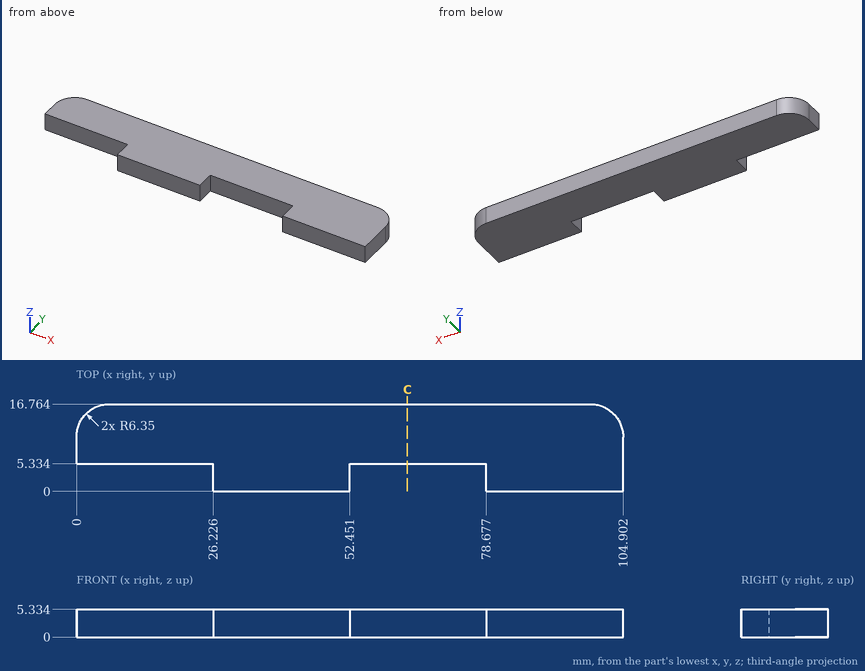
Geometry check sheet. Reference: drawing and pictorial views, mm from the part's lowest x, y, z. Round coordinates to 2 decimals unless told otherwise and drop trailing zeros. Order: outer loops, then holes, each group sorted by start corner. A loop starts at its lowest first (then second) coordinate and runs counter-clockwise, first axis right, second up. Notation, with made-up numbers: (-38.75, -33) - (-33.75, -33) arc R22 cw to (-33.75, -22) - close; hole circle Ø5 at (79.5, -6). An arc over 180 degrees is marked (long way). Use a Markdown table: item, result. Add a question column.
1) Gauge pin test, flat ends, axial feed: P1, Ø2, axis at x = 74.5, z = 1.5, coming from the -Y side; P2, Ø2, axis at y = 14, z = 4, coming from the +X side; P3, Ø2.5, axis at y = 2.5, z = 2.5, coming from the -X side (1 decimal). Record the tip position at first contact, or that the pin passes through.
2) Thickness scan on line 1 along Y through (x, z) = (76.5, 4.6) (1 decimal); line 2 along X through (y, z) = (15.25, 4.7) (1 decimal); line 3 along Y through (x, z) = (5.5, 4.2) (1 decimal). Record the ranges inside material, lowest first.
3) Section check C-C (x = 63.5). Record the cut outline in (y, z) (1 decimal).
Established:
| question | item | result |
|---|---|---|
| 1 | P1 | y = 5.33 |
| 1 | P2 | x = 104.35 |
| 1 | P3 | x = 26.2 |
| 2 | line 1 | 5.3 to 16.8 |
| 2 | line 2 | 2.2 to 102.7 |
| 2 | line 3 | 5.3 to 16.7 |
| 3 | outline | (5.3, 0) - (16.8, 0) - (16.8, 5.3) - (5.3, 5.3) - close |
